```python
from build123d import *

# Parameters (mm, degrees)
SKETCH1_R           = 2.75
BOSS_EXTRUDE1_DEPTH = 3.125


with BuildPart() as part:
    # Sketch1 → Boss-Extrude1 (new body)
    with BuildSketch(Plane.XY):
        with BuildLine():
            Line((-32.5, 20), (32.5, 20))
            Line((32.5, 20), (62.377876431, -31.75))
            Line((62.377876431, -31.75), (32.5, -31.75))
            Line((32.5, -31.75), (5, -31.75))
            Line((5, -31.75), (5, 0))
            ThreePointArc((5, 0), (0, 5), (-5, 0))
            Line((-5, 0), (-5, -31.75))
            Line((-5, -31.75), (-32.5, -31.75))
            Line((-32.5, -31.75), (-32.5, 20))
        make_face()
        with Locations((0, 12.125)):
            Circle(SKETCH1_R, mode=Mode.SUBTRACT)
    extrude(amount=BOSS_EXTRUDE1_DEPTH)


solid = part.part
```
CAD build for the part. Positions are in the model's coordinates, mm. A direction names the side the tool comes from. Coordinates: 2 decimals unless noted, no trailing zeros. Order: outer loops, then holes, each group sorted by start corner. A loop starts at its lowest first (then second) coordinate and runs counter-clockwise, first axis right, second up. Notation, with made-up numbers: (-2, 33.25) -> (23, 33.25) arc R29 ccw to (23, 54.25) -> close; hole circle Ø1 at (80.25, 36.5). An arc over 180 degrees is marked (long way). Use one line per item in the form item = value. Start each with the question number.
1) Band-saw the part on A-A on x = 0. Give the cut face in (y, z) (3 decimals).
2) Pull direction X, two halves, no side cores. Call faces 1 (the flat face through (47.23, -5.51, 1.54)), 2 (the flat face through (-5, -16, 2)), 3 (the flat face through (0, 20, 2)): +X half, -X half, draft (parallel to the pull), parting line (faces both ways), or undercut.
3) Drill centre lines: L1, parallel to Y at x = 0, z = 1.9 (3 decimals); L2, parallel to X at y = -14, z = 1.3; L3, parallel to X at y = 10, z = 0.5. Where is each one in solid material? Low to high. Write a range as [from, to].
4) Tool access for faces 4 (the flat face through (-19, -31.75, 2)), 5 (the flat face through (5, -16, 2)): list every direction of +Z, -Z, +X, -X, +Y, -Y with a clear straight run to the whole face (end or side of a thin tool).
5) Band-saw the part on D-D on x = 52.5. Give the cut face in (y, z) (3 decimals).
6) Band-saw the part on B-B on y = -17. Give the cut face in (x, z) (3 decimals), then the cut area to 3 significant figures.
7) Band-saw the part on C-C on z = 1.2. Give the cut face in (x, y) (3 decimals), then the cut area to 3 significant figures.
Entries:
q1.outline = (5, 0) -> (9.375, 0) -> (9.375, 3.125) -> (5, 3.125) -> close; (14.875, 0) -> (20, 0) -> (20, 3.125) -> (14.875, 3.125) -> close
q2.face_1 = +X half
q2.face_2 = undercut
q2.face_3 = draft
q3.L1 = [5, 9.375], [14.875, 20]
q3.L2 = [-32.5, -5], [5, 52.13]
q3.L3 = [-32.5, -1.75], [1.75, 38.27]
q4.face_4 = +Z, -Z, +X, -X, -Y
q4.face_5 = +Z, -Z, -Y
q5.outline = (-31.75, 0) -> (-14.641, 0) -> (-14.641, 3.125) -> (-31.75, 3.125) -> close
q6.outline = (-32.5, 0) -> (-5, 0) -> (-5, 3.125) -> (-32.5, 3.125) -> close; (5, 0) -> (53.862, 0) -> (53.862, 3.125) -> (5, 3.125) -> close
q6.area = 239 mm2
q7.outline = (-32.5, -31.75) -> (-5, -31.75) -> (-5, 0) arc R5 cw to (5, 0) -> (5, -31.75) -> (62.378, -31.75) -> (32.5, 20) -> (-32.5, 20) -> close; hole circle Ø5.5 at (0, 12.125)
q7.area = 3,760 mm2
